Geometry: final body of the model. Coordinates: model frame, mm. Coordinates: 2 decimals unless noted, no trailing zeros. Order: outer loops, then holes, each group sorted by start corner. A loop starts at its lowest first (then second) coordinate and runs counter-clockwise, first axis right, second up. Notation, with made-up numbers: M -38.5,-19 L -16.5,-19 A16 cw -16.5,3 Z; hole C 57.25,74.25 d9. An arc over 180 degrees is marked long. Use CSV: the item, a comma, the result in double quotes. Start each with the question number.
1. First-contact query: P1, Ø5, axis at x = 10, z = -111.5, coming from the +Y side; P2, Ø4.5, axis at x = -3.81, z = -173.355, coming from the -Y side; P3, Ø1.3, axis at y = 1, z = -81, coming from the -X side. Flat tips, straight axial feed; report the tip coordinate or a pass-through.
2. Section query A-A on z = -54.5. Return the cut outline in (x, y).
3. Section query B-B on y = 1.9. Return the cut outline in (x, z) (3 decimals).
4. Material intervals for line 1 (Z direction, x = 9, y = 1.15); line 2 (X direction, y = 1, z = -163); line 3 (Z direction, x = 7.5, y = 1.35), sorted ascending.
from build123d import *

# Parameters (mm, degrees)
SKETCH1_R           = 1.651
BOSS_EXTRUDE1_DEPTH = 2.54


with BuildPart() as part:
    # Sketch1 → Boss-Extrude1 (new body)
    with BuildSketch(Plane(origin=(0, 0, 0), x_dir=(1, 0, 0), z_dir=(0, 1, 0))):
        with BuildLine():
            Line((0, 0), (5.08, 0))
            Line((5.08, 0), (5.08, 165.1))
            ThreePointArc((5.08, 165.1), (6.195923164, 167.794076836), (8.89, 168.91))
            ThreePointArc((8.89, 168.91), (13.335, 173.355), (8.89, 177.8))
            Line((8.89, 177.8), (-3.81, 177.8))
            ThreePointArc((-3.81, 177.8), (-8.255, 173.355), (-3.81, 168.91))
            ThreePointArc((-3.81, 168.91), (-1.115923164, 167.794076836), (0, 165.1))
            Line((0, 165.1), (0, 0))
        make_face()
        with Locations((-3.81, 173.355)):
            Circle(SKETCH1_R, mode=Mode.SUBTRACT)
        with Locations((8.89, 173.355)):
            Circle(SKETCH1_R, mode=Mode.SUBTRACT)
    extrude(amount=BOSS_EXTRUDE1_DEPTH)


solid = part.part
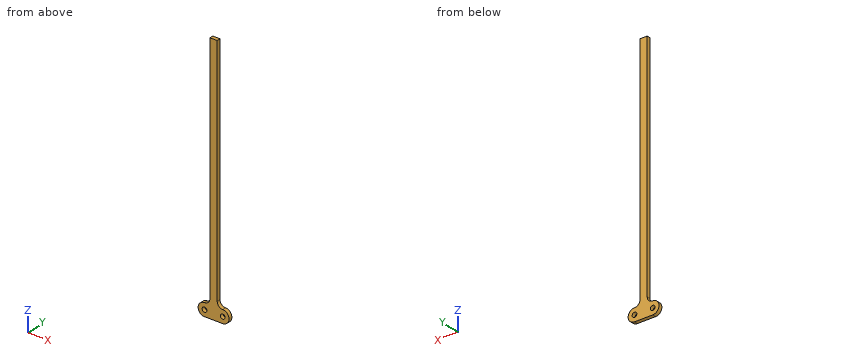
Results list:
1,P1,"passes through"
1,P2,"stops at y = 0"
1,P3,"stops at x = 0"
2,outline,"M 0,0 L 5.08,0 L 5.08,2.54 L 0,2.54 Z"
3,outline,"M -3.81,-177.8 L 8.89,-177.8 A4.445 ccw 8.89,-168.91 A3.81 cw 5.08,-165.1 L 5.08,0 L 0,0 L 0,-165.1 A3.81 cw -3.81,-168.91 A4.445 ccw Z; hole C -3.81,-173.355 d3.302; hole C 8.89,-173.355 d3.302"
4,line 1,"z = -177.8 to -175, -171.71 to -168.91"
4,line 2,"x = 0 to 5.08"
4,line 3,"z = -177.8 to -174.25, -172.46 to -168.65"
